```python
from build123d import *
from build123d.topology import SkipClean

# Parameters (mm, degrees)
SKETCH_1_R      = 1
EXTRUDE_1_DEPTH = 5
EXTRUDE_2_DEPTH = 5


with BuildPart() as part:
    # 草图1 → 凸台-拉伸1 (new body)
    with BuildSketch(Plane.XY):
        with Locations((-12.637856913, 12.301005314)):
            Circle(SKETCH_1_R)
    extrude(amount=EXTRUDE_1_DEPTH)

    # 草图2 → 凸台-拉伸2 (add)
    with SkipClean():  # the faces are left unmerged after this step: merging them gives an invalid solid
        with BuildSketch(Plane.XY.offset(5)):
            with BuildLine():
                Line((-13.503882317, 12.801005314), (-11.771831509, 12.801005314))
                ThreePointArc((-11.771831509, 12.801005314), (-11.637856913, 12.301005314), (-11.771831509, 11.801005314))
                Line((-11.771831509, 11.801005314), (-13.503882317, 11.801005314))
                ThreePointArc((-13.503882317, 11.801005314), (-13.637856913, 12.301005314), (-13.503882317, 12.801005314))
            make_face()
        extrude(amount=EXTRUDE_2_DEPTH)


solid = part.part
```
CAD build for the part. Positions are in the model's coordinates, mm. A direction names the side the tool comes from. Give positions to 0.01 mm unless a question says otherwise; leave off trailing zeros. Order: outer loops, then holes, each group sorted by start corner. A loop starts at its lowest first (then second) coordinate and runs counter-clockwise, first axis right, second up.
(1) Tool access for faces 1 (the flat face through (-13, 12, 0)), 2 (the flat face through (-13, 11.801, 7)), 3 (the flat face through (-13, 12.801, 7)): list every direction of +Z, -Z, +X, -X, +Y, -Y with a clear straight run to the whole face (end or side of a thin tool).
(2) Saw through at A-A, the plane x = -12.25. Give the cut face in (y, z).
(3) Saw through at B-B, the plane z = 6. Give the cut face in (x, y).
(4) Flat gauge pins, fed straight in: pin 1 (1 mm diameter, centred on x = -12.5, y = 12, fed in from -Z); pin 2 (0.5 mm diameter, centred on x = -12.5, z = 8.5, fed in from +Y); pin 3 (0.9 mm diameter, centred on x = -12.5, z = 6.5, fed in from -Y). Where does each tip first touch, or does it go through?
(5) Saw through at C-C, the plane y = 12.6. Give the cut face in (x, z).
(6) Saw through at D-D, the plane x = -12.7. Give the cut face in (y, z).
(7) Drill centre lines: L1, parallel to Y at x = -11.95, z = 7; L2, parallel to Z at x = -13.25, y = 11.6; L3, parallel to X at y = 12.2, z = 6.5. Where is each one in solid material? Low to high.
Results found:
1. face 1: -Z, +X, -X, +Y, -Y
1. face 2: +Z, +X, -X, -Y
1. face 3: +Z, +X, -X, +Y
2. outline: (11.38, 0) - (13.22, 0) - (13.22, 5) - (12.8, 5) - (12.8, 10) - (11.8, 10) - (11.8, 5) - (11.38, 5) - close
3. outline: (-13.5, 11.8) - (-11.77, 11.8) arc R1 ccw to (-11.77, 12.8) - (-13.5, 12.8) arc R1 ccw to start
4. pin 1: stops at z = 0
4. pin 2: stops at y = 12.8
4. pin 3: stops at y = 11.8
5. outline: (-13.59, 0) - (-11.68, 0) - (-11.68, 10) - (-13.59, 10) - close
6. outline: (11.3, 0) - (13.3, 0) - (13.3, 5) - (12.8, 5) - (12.8, 10) - (11.8, 10) - (11.8, 5) - (11.3, 5) - close
7. L1: y = 11.8 to 12.8
7. L2: z = 0 to 5
7. L3: x = -13.63 to -11.64
